```python
from build123d import *

# Parameters (mm, degrees)
SKETCH1_W           = 1200
SKETCH1_H           = 600
BOSS_EXTRUDE1_DEPTH = 25
SKETCH2_W           = 40
SKETCH2_H           = 40
BOSS_EXTRUDE2_DEPTH = 750
FILLET1_R           = 3


with BuildPart() as part:
    # Sketch1 → Boss-Extrude1 (new body)
    with BuildSketch(Plane.XY):
        Rectangle(SKETCH1_W, SKETCH1_H)
    extrude(amount=BOSS_EXTRUDE1_DEPTH)

    # Sketch2 → Boss-Extrude2 (add)
    with BuildSketch(Plane.XY):
        with Locations((-560, 260)):
            Rectangle(SKETCH2_W, SKETCH2_H)
        with Locations((560, 260)):
            Rectangle(SKETCH2_W, SKETCH2_H)
        with Locations((-560, -260)):
            Rectangle(SKETCH2_W, SKETCH2_H)
        with Locations((560, -260)):
            Rectangle(SKETCH2_W, SKETCH2_H)
    extrude(amount=-BOSS_EXTRUDE2_DEPTH)

    # Fillet1
    fillet1_edges = [part.edges().sort_by_distance(p)[0] for p in [
        (-600, 0, 25),
        (0, -300, 25),
        (580, 280, -375),
        (580, 240, -375),
        (540, 280, -375),
        (-540, -240, -375),
        (-580, -280, -375),
        (-580, -240, -375),
        (580, -240, -375),
        (580, -280, -375),
        (540, -240, -375),
        (-540, 280, -375),
        (-540, 240, -375),
        (-580, 280, -375),
        (600, 0, 25),
        (0, 300, 25),
    ]]
    fillet(fillet1_edges, radius=FILLET1_R)


solid = part.part
```
The listing builds one solid part. Answer for the finished solid, in the listing's coordinates (mm). A direction names the side the tool comes from. Round coordinates to 2 decimals unless told otherwise and drop trailing zeros. Loops run counter-clockwise (first coordinate to the right, second up) from the corner with the lowest first, then second, coordinate; pieces in that order, holes last.
Q1. Section B-B, the plane x = 217.5 is taken. Determine the outline of the cut face in (y, z), then the cut area to 3 significant figures.
Q2. For a pull along Y with two mould halves and no side action, classify faces 4 (the face through (558, 240, -370)), 5 (the face through (540, 258, -370)), 6 (the face through (560, 280, -370)), 7 (the face through (558, -280, -370)) as released by +Y, released by -Y, zero draft, split by the parting line, or undercut.
Q3. Find the intervals of material crossed by line 1 (X direction, y = -249.5, z = -113.5); line 2 (Y direction, x = 547, z = -276.5); line 3 (Z direction, x = -279, y = 238), in increasing order.
Q4. Given pin 1 Ø5 at (x, y) = (-258, 238) entering from -Z; pin 2 Ø18.5 at (x, z) = (-561.5, -206) entering from -Y; pin 3 Ø17 at (y, z) = (-259, -453) entering from +X, each flat-ended and moving along its own axis, determine where each tip first touches the part or whether it passes through.
Q5. Section A-A, the plane z = -428 is taken. Determine the outline of the cut face in (x, y).
Q6. Which of the six approach directions +Z, -Z, +X, -X, +Y, -Y give full straight-line access (tool end or side, diameter ignored) to faces 1 (the face through (-540, 260, -370)), 2 (the face through (-559, -280, -370)), 3 (the face through (-562, 240, -370))?
Q7. Section C-C, the plane y = -36 is taken. Determine the outline of the cut face in (x, z), then the cut area to 3 significant figures.
Completed:
1. outline: (-300, 0) - (300, 0) - (300, 22) arc R3 ccw to (297, 25) - (-297, 25) arc R3 ccw to (-300, 22) - close
1. area: 15,000 mm2
2. face 4: undercut
2. face 5: zero draft
2. face 6: released by +Y
2. face 7: released by -Y
3. line 1: x = -580 to -540, 540 to 580
3. line 2: y = -280 to -240, 240 to 280
3. line 3: z = 0 to 25
4. pin 1: stops at z = 0
4. pin 2: stops at y = -280
4. pin 3: stops at x = 580
5. outline: (-580, -277) arc R3 ccw to (-577, -280) - (-540, -280) - (-540, -243) arc R3 ccw to (-543, -240) - (-577, -240) arc R3 ccw to (-580, -243) - close; (-580, 240) - (-543, 240) arc R3 ccw to (-540, 243) - (-540, 277) arc R3 ccw to (-543, 280) - (-577, 280) arc R3 ccw to (-580, 277) - close; (540, -280) - (577, -280) arc R3 ccw to (580, -277) - (580, -243) arc R3 ccw to (577, -240) - (543, -240) arc R3 ccw to (540, -243) - close; (540, 240) - (577, 240) arc R3 ccw to (580, 243) - (580, 277) arc R3 ccw to (577, 280) - (543, 280) arc R3 ccw to (540, 277) - close
6. face 1: -Z, +Y, -Y
6. face 2: -Z, +X, -X, -Y
6. face 3: -Z, +X, -X
7. outline: (-600, 0) - (600, 0) - (600, 22) arc R3 ccw to (597, 25) - (-597, 25) arc R3 ccw to (-600, 22) - close
7. area: 30,000 mm2
